Can you work these out from the model? Positions are in its coordinate system, mm. A direction names the side the tool comes from. Coordinates: 2 decimals unless noted, no trailing zeros. Loops run counter-clockwise (first coordinate to the right, second up) from the corner with the lowest first, then second, coordinate; pieces in that order, holes last. Notation, with made-up numbers: (16.5, 74.25) -> (40.5, 74.25) arc R7 cw to (40.5, 82.25) -> close; hole circle Ø10 at (8.5, 55). An arc over 180 degrees is marked (long way). Put each result on its own line as item: value. Start each with the question number.
Item 1: If we section it at A-A on y = 13.5: Please give me the cut outline in (x, z), plus the area to 3 significant figures.
Item 2: If we section it at B-B on x = -6.4: Please give me the cut outline in (y, z), plus the area to 3 significant figures.
Item 3: Please list where these lines run through material, in increasing order: L1, parallel to Y at x = 6.4, z = 0.85; L2, parallel to Y at x = -5.5, z = 0.8; L3, parallel to X at y = -12, z = 1. Write a range as from..to.
Item 4: If we section it at D-D on x = 9: Please give me the cut outline in (y, z).
Item 5: If we section it at C-C on z = 0.3: Please give me the cut outline in (x, y).
Item 6: For faces 4 (the cylindrical face through (9.8, -9, 0.6)), 5 (the cylindrical face through (-5, -13, 1)), which set-ups out of +Z, -Z, +X, -X, +Y, -Y let a thin tool reach every point of the face, with its end or its side?
Item 7: We'd pull the mould along X, two halves only. Please class faces 1 (the cylindrical face through (0.59, 16.64, 0.59)), 2 (the flat face through (6, 13, 1.2)), 3 (the cylindrical face through (5, -13, 1)): pulls with the +X half, pulls with the -X half, needs draft (parallel to the pull), parting line crosses it, or undercut.
```python
from build123d import *

# Parameters (mm, degrees)
SKETCH1_R  = 1
BODY_DEPTH = 1.2


with BuildPart() as part:
    # Sketch1 → Body (new body)
    with BuildSketch(Plane.XY):
        with BuildLine():
            Line((4.139124405, -11.62116667), (4.293680087, -12.055103216))
            ThreePointArc((4.293680087, -12.055103216), (5.433429283, -13.240393983), (7.076323895, -13.170825851))
            ThreePointArc((7.076323895, -13.170825851), (0, 16.65), (-7.076323895, -13.170825851))
            ThreePointArc((-7.076323895, -13.170825851), (-5.433429283, -13.240393983), (-4.293680087, -12.055103216))
            Line((-4.293680087, -12.055103216), (-4.139124405, -11.62116667))
            ThreePointArc((-4.139124405, -11.62116667), (-4.850462528, -8.983168612), (-7.570021573, -8.720424866))
            ThreePointArc((-7.570021573, -8.720424866), (-9.727430565, -9.019484739), (-11.518571073, -7.780264805))
            ThreePointArc((-11.518571073, -7.780264805), (0, 13.9), (11.518571073, -7.780264805))
            ThreePointArc((11.518571073, -7.780264805), (9.727430565, -9.019484739), (7.570021573, -8.720424866))
            ThreePointArc((7.570021573, -8.720424866), (4.850462528, -8.983168612), (4.139124405, -11.62116667))
        make_face()
        with Locations((-6.4, -10.815907989)):
            Circle(SKETCH1_R, mode=Mode.SUBTRACT)
        with Locations(Location((6.4, -10.815907989, 0), (0, 0, 180))):
            Circle(SKETCH1_R, mode=Mode.SUBTRACT)
    extrude(amount=BODY_DEPTH)


solid = part.part
```
Solutions:
1. outline: (-9.45, 0) -> (-3.31, 0) -> (-3.31, 1.2) -> (-9.45, 1.2) -> close; (3.31, 0) -> (9.45, 0) -> (9.45, 1.2) -> (3.31, 1.2) -> close
1. area: 14.7 mm^2
2. outline: (-13.37, 0) -> (-11.82, 0) -> (-11.82, 1.2) -> (-13.37, 1.2) -> close; (-9.82, 0) -> (-8.42, 0) -> (-8.42, 1.2) -> (-9.82, 1.2) -> close; (12.34, 0) -> (15.29, 0) -> (15.29, 1.2) -> (12.34, 1.2) -> close
2. area: 7.09 mm^2
3. L1: -13.37..-11.82, -9.82..-8.42, 12.34..15.29
3. L2: -13.27..-11.25, -10.38..-8.59, 12.77..15.66
3. L3: -9.04..-4.27, 4.27..9.04
4. outline: (-12.03, 0) -> (-9.1, 0) -> (-9.1, 1.2) -> (-12.03, 1.2) -> close; (10.59, 0) -> (13.83, 0) -> (13.83, 1.2) -> (10.59, 1.2) -> close
5. outline: (-11.52, -7.78) arc R13.9 cw (long way) to (11.52, -7.78) arc R3 cw to (7.57, -8.72) arc R2.4 ccw to (4.14, -11.62) -> (4.29, -12.06) arc R2 ccw to (7.08, -13.17) arc R15.75 ccw (long way) to (-7.08, -13.17) arc R2 ccw to (-4.29, -12.06) -> (-4.14, -11.62) arc R2.4 ccw to (-7.57, -8.72) arc R3 cw to start; hole circle Ø2 at (-6.4, -10.82); hole circle Ø2 at (6.4, -10.82)
6. face 4: +Z, -Z
6. face 5: +Z, -Z, -Y
7. face 1: parting line crosses it
7. face 2: needs draft
7. face 3: undercut
